Input: dimensioned drawing with shaded views. Units: mm. Origin: part minimum x, y, z. A direction names the side the tool comes from. Round coordinates to 2 decimals unless told otherwise and drop trailing zeros. Order: outer loops, then holes, each group sorted by start corner. A loop starts at its lowest first (then second) coordinate and runs counter-clockwise, first axis right, second up.
Item 1: Cut plane C-C on x = 14. Output: boundary loops of the cut face in (y, z).
Item 2: First-contact query: pin 1 (3 mm diameter, centred on x = 9.5, z = 19.5, fed in from -Y); pin 2 (3.5 mm diameter, centred on y = 10, z = 52, fed in from +X); pin 3 (5 mm diameter, centred on x = 9, y = 28.5, fed in from -Z). Flat tips, straight axial feed; report the tip coordinate or a pass-through.
Item 3: Cut plane D-D on y = 36. Output: boundary loops of the cut face in (x, z), then the cut area to 3 significant figures.
Item 4: Reachability of the marked faces 1 and 2 from +Z, -Z, +X, -X, +Y, -Y: full face, straight path, thin tool, end or side. Return the list, or none.
Item 5: Cut plane A-A on z = 10. Output: boundary loops of the cut face in (x, y), then the cut area to 3 significant figures.
Item 6: Line query: L1, parallel to Y at x = 4.5, z = 52; L2, parallel to Y at x = 4.25, z = 30; L3, parallel to Y at x = 1.25, z = 17. Output: solid intervals per line, ascending.
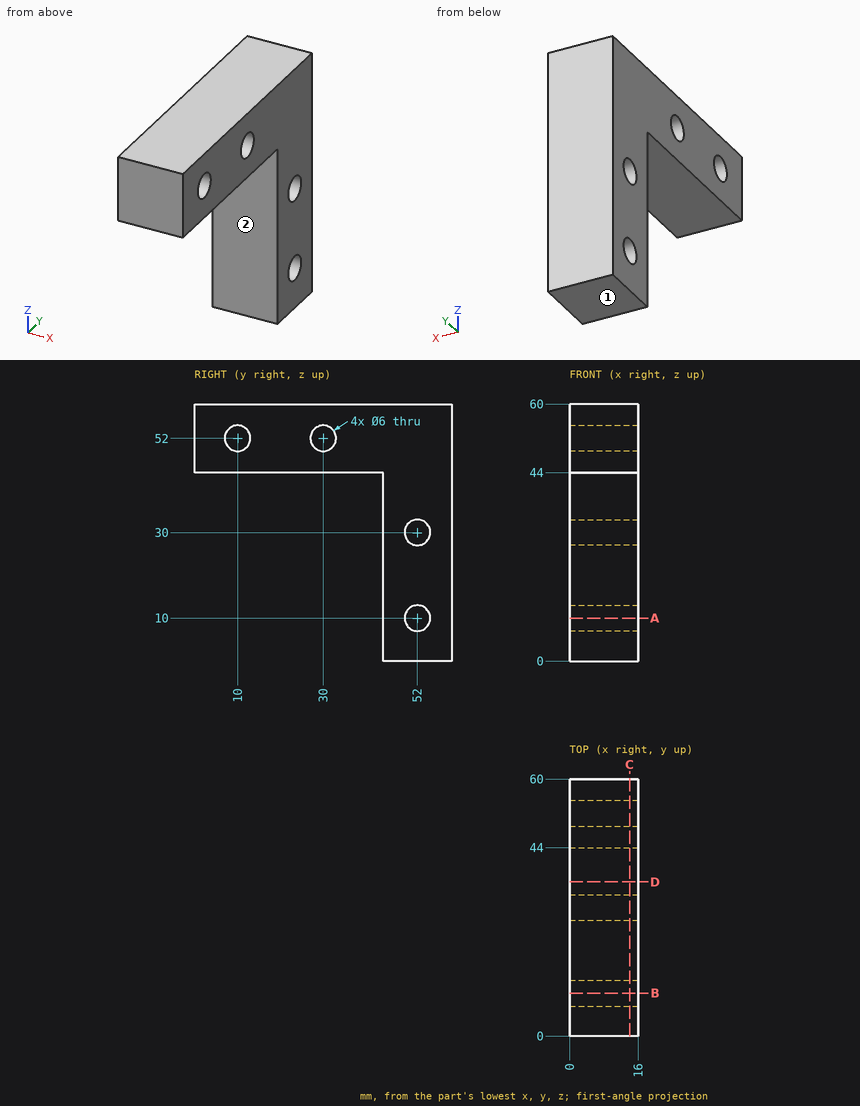
From the geometry:
1. outline: (0, 44) - (44, 44) - (44, 0) - (60, 0) - (60, 60) - (0, 60) - close; hole circle Ø6 at (10, 52); hole circle Ø6 at (30, 52); hole circle Ø6 at (52, 10); hole circle Ø6 at (52, 30)
2. pin 1: stops at y = 44
2. pin 2: passes through
2. pin 3: stops at z = 44
3. outline: (0, 44) - (16, 44) - (16, 60) - (0, 60) - close
3. area: 256 mm2
4. face 1: -Z, +X, -X, +Y, -Y
4. face 2: -Z, +X, -X, -Y
5. outline: (0, 44) - (16, 44) - (16, 49) - (0, 49) - close; (0, 55) - (16, 55) - (16, 60) - (0, 60) - close
5. area: 160 mm2
6. L1: y = 0 to 7, 13 to 27, 33 to 60
6. L2: y = 44 to 49, 55 to 60
6. L3: y = 44 to 60
